Geometry: final body of the model. Coordinates: model frame, mm. Face numbers are marked on the shaded views. A direction names the side the tool comes from. Round coordinates to 2 decimals unless told otherwise and drop trailing zeros. Write each loop counter-clockwise with the first axis right and the second up, starting at its lowest first coordinate (ties: lowest second). Pieces come first, ordered by that corner, then holes. Notation, with made-up numbers: (54, 32) - (59, 32) arc R6 cw to (59, 38) - close; hole circle Ø10 at (24, 82.25). An arc over 180 degrees is marked (long way). Write each question's results on one line, items separated by ' | '.
from build123d import *

# Parameters (mm, degrees)
PAD_DEPTH       = 20
SKETCH001_W     = 9
SKETCH001_H     = 6
POCKET_DEPTH    = 8
SKETCH002_W     = 4.2
SKETCH002_H     = 4.2
POCKET001_DEPTH = 5


with BuildPart() as part:
    # Sketch → Pad (new body)
    with BuildSketch(Plane.YZ):
        Polygon((-27.098937, -22.548221), (27.401063, -22.548221), (27.401063, 8.451779), (20.651063, 8.451779), (20.651063, -19.548221), (-20.348937, -19.548221), (-20.348937, 8.451779), (-27.098937, 8.451779), align=None)
    extrude(amount=PAD_DEPTH)

    # Sketch001 → Pocket (cut)
    with BuildSketch(Plane(origin=(0, 27.401063, 0), x_dir=(-1, 0, 0), z_dir=(0, 1, 0))):
        with Locations((-9.865053, -13.762334)):
            Rectangle(SKETCH001_W, SKETCH001_H)
    extrude(amount=-POCKET_DEPTH, mode=Mode.SUBTRACT)

    # Sketch002 (on Face4 of Pocket) → Pocket001 (cut)
    with BuildSketch(Plane(origin=(0, 0, 0), x_dir=(0, 1, 0), z_dir=(-1, 0, 0))):
        with Locations((-23.796906, 18.893097)):
            Rectangle(SKETCH002_W, SKETCH002_H)
        with Locations((23.941537, 18.893097)):
            Rectangle(SKETCH002_W, SKETCH002_H)
    extrude(amount=-POCKET001_DEPTH, mode=Mode.SUBTRACT)


solid = part.part
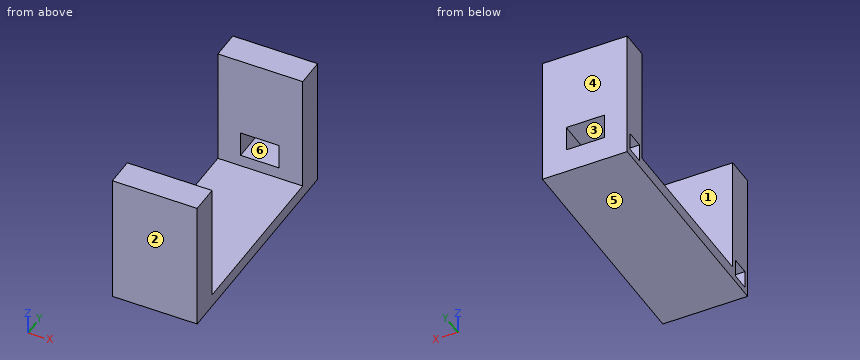
Q1. Section query A-A, the plane x = 11. Return loops of the section in (y, z).
Answer block:
outline: (-27.1, -22.55) - (27.4, -22.55) - (27.4, -16.76) - (20.65, -16.76) - (20.65, -19.55) - (-20.35, -19.55) - (-20.35, 8.45) - (-27.1, 8.45) - close; (20.65, -10.76) - (27.4, -10.76) - (27.4, 8.45) - (20.65, 8.45) - close
Q2. Ray query, line 1 along Z through (x, y) = (4.5, 23.5); line 2 along Y through (x, z) = (18.75, -15.5); line 3 along X through (y, z) = (22.5, -16). Return the intervals inside material, ascending.
Answer block:
line 1: -22.55 to -20.99, -16.79 to 8.45 | line 2: -27.1 to -20.35, 20.65 to 27.4 | line 3: 0 to 5.37, 14.37 to 20
Q3. Section query C-C, the plane z = 3. Return loops of the section in (x, y).
Answer block:
outline: (0, -27.1) - (20, -27.1) - (20, -20.35) - (0, -20.35) - close; (0, 20.65) - (20, 20.65) - (20, 27.4) - (0, 27.4) - close
Q4. Section query B-B, the plane z = -12. Return loops of the section in (x, y), plus the area to 3 significant figures.
Answer block:
outline: (0, -27.1) - (20, -27.1) - (20, -20.35) - (0, -20.35) - close; (0, 20.65) - (5.37, 20.65) - (5.37, 27.4) - (0, 27.4) - close; (14.37, 20.65) - (20, 20.65) - (20, 27.4) - (14.37, 27.4) - close | area: 209 mm2
Q5. Access query for the marked faces 1 and 2. Directions: +Z, -Z, +X, -X, +Y, -Y. A direction counts if a zero-diameter tool reaches every point of the face in a straight line with its end or side. Return the directions, or none.
Answer block:
face 1: +Z, +X, -X | face 2: +Z, -Z, +X, -X, -Y
Q6. Mould query, pull axis Z, two halves, no side actions, for the marked faces 3, 4, 5 and 6. Classes: pulls with the +Z half, pulls with the -Z half, needs draft (parallel to the pull), parting line crosses it, or undercut.
Answer block:
face 3: undercut | face 4: needs draft | face 5: pulls with the -Z half | face 6: undercut
Q7. Pin query (flat end, axial travel): pin 1 (6 mm diameter, centred on y = -2, z = -16, fed in from +X); pin 2 (1.3 mm diameter, centred on y = -24.5, z = -19.5, fed in from -X); pin 3 (3.5 mm diameter, centred on y = 24, z = -18.5, fed in from -X); pin 4 (2 mm diameter, centred on x = 2.5, y = 16.5, fed in from +Z). Return the tip coordinate at first contact, or that it passes through.
Answer block:
pin 1: through | pin 2: x = 5 | pin 3: x = 0 | pin 4: z = -19.55
Q8. Section query D-D, the plane x = 4.25. Return loops of the section in (y, z), plus the area to 3 significant figures.
Answer block:
outline: (-27.1, -22.55) - (27.4, -22.55) - (27.4, 8.45) - (20.65, 8.45) - (20.65, -19.55) - (-20.35, -19.55) - (-20.35, 8.45) - (-27.1, 8.45) - close; hole (-25.9, -20.99) - (-21.7, -20.99) - (-21.7, -16.79) - (-25.9, -16.79) - close; hole (21.84, -20.99) - (26.04, -20.99) - (26.04, -16.79) - (21.84, -16.79) - close | area: 506 mm2
